```python
from build123d import *

# Parameters (mm, degrees)
SKETCH2_W           = 15
SKETCH2_H           = 16
BOSS_EXTRUDE2_DEPTH = 25
SKETCH3_R           = 2.5
BOSS_EXTRUDE3_DEPTH = 5
CHAMFER1_SIZE       = 12.5
CHAMFER1_SIZE2      = 3.349364905
CHAMFER2_SIZE       = 12.5
CHAMFER2_SIZE_2     = 3.349364905


with BuildPart() as part:
    # Sketch2 → Boss-Extrude2 (new body)
    with BuildSketch(Plane.XY):
        with Locations((7.5, 8)):
            Rectangle(SKETCH2_W, SKETCH2_H)
    extrude(amount=BOSS_EXTRUDE2_DEPTH)

    # Sketch3 → Boss-Extrude3 (add)
    with BuildSketch(Plane.ZY):
        with Locations(Location((5.5, 7.837863741, 0), (0, 0, 90))):
            Circle(SKETCH3_R)
        with Locations(Location((19.5, 7.837863741, 0), (0, 0, 90))):
            Circle(SKETCH3_R)
    extrude(amount=BOSS_EXTRUDE3_DEPTH)

    # Chamfer1
    chamfer1_edges = [part.edges().sort_by_distance(p)[0] for p in [
        (7.5, 0, 25),
    ]]
    chamfer1_side = [part.faces().sort_by_distance(p)[0] for p in [
        (7.5, 0, 12.5),
    ]]
    chamfer(chamfer1_edges, length=CHAMFER1_SIZE, length2=CHAMFER1_SIZE2, reference=chamfer1_side[0])

    # Chamfer2
    # the kernel refuses this chamfer: 12.5, 3.349364905 mm, written as the material it takes off along each edge
    with BuildSketch(Plane(origin=(-32.459019628, 0, 0), x_dir=(0, -0.009967146577156423, 0.9999503267608394), z_dir=(1, 0, 0))) as chamfer2_piece_1:
        Polygon((CHAMFER2_SIZE * 0.999950326761, -CHAMFER2_SIZE * 0.00996714657716), (-CHAMFER2_SIZE_2 * 0.00996714657831, -CHAMFER2_SIZE_2 * 0.999950326877), (0, 0), align=None)
    extrude(amount=79.918039255, mode=Mode.SUBTRACT)


solid = part.part
```
Input: part model. Units: mm. Frame: model coordinates. A direction names the side the tool comes from. Round coordinates to 2 decimals unless told otherwise and drop trailing zeros. Loops run counter-clockwise (first coordinate to the right, second up) from the corner with the lowest first, then second, coordinate; pieces in that order, holes last.
1) Section query D-D on z = 5.5. Return the cut outline in (x, y), plus the area to 3 significant figures.
Ans:
outline: (-5, 5.34) - (0, 5.34) - (0, 1.88) - (15, 1.88) - (15, 16) - (0, 16) - (0, 10.34) - (-5, 10.34) - close
area: 237 mm2
2) Pin query (flat end, axial travel): pin 1 (1 mm diameter, centred on y = 13, z = 7.5, fed in from -X). Return the tip coordinate at first contact, or that it passes through.
Ans:
pin 1: stops at x = 0
3) Section query A-A on x = -1.5. Return the cut outline in (y, z), plus the area to 3 significant figures.
Ans:
outline: circle Ø5 at (7.84, 5.5); circle Ø5 at (7.84, 19.5)
area: 39.3 mm2
4) Section query C-C on y = 7.75. Return the cut outline in (x, z).
Ans:
outline: (-5, 3) - (0, 3) - (0, 0) - (15, 0) - (15, 25) - (0, 25) - (0, 22) - (-5, 22) - (-5, 17) - (0, 17) - (0, 8) - (-5, 8) - close
5) Pull-direction query (Z, two-part tool) for faces 3 (the flat face through (-5, 8, 19)), 4 (the flat face through (7, 10, 0)), 5 (the cylindrical face through (-2.46, 5.34, 5.39)); classes: released by +Z, released by -Z, zero draft, split by the parting line, or undercut.
Ans:
face 3: zero draft
face 4: released by -Z
face 5: undercut
6) Material intervals for line 1 (X direction, y = 8.75, z = 16.5); line 2 (Z direction, x = -2, y = 7.25); line 3 (Y direction, x = 8.75, z = 20.25), sorted ascending.
Ans:
line 1: x = 0 to 15
line 2: z = 3.07 to 7.93, 17.07 to 21.93
line 3: y = 2.08 to 16
7) Section query B-B on x = 11.5. Return the cut outline in (y, z), plus the area to 3 significant figures.
Ans:
outline: (0, 12.5) - (3.35, 0) - (16, 0) - (16, 25) - (3.35, 25) - close
area: 358 mm2
8) Set-up query: faces 1 (the cylindrical face through (-2.465, 5.995, 17.81)), 2 (the flat face through (15, 8, 12)). Return all of +Z, -Z, +X, -X, +Y, -Y with unobstructed straight access to the full face (end or side cutting, diameter ignored); none if empty.
Ans:
face 1: -X
face 2: +Z, -Z, +X, +Y, -Y
